The listing builds one solid part. Answer for the finished solid, in the listing's coordinates (mm). A direction names the side the tool comes from. Give positions to 0.01 mm unless a question says otherwise; leave off trailing zeros. Order: outer loops, then holes, each group sorted by start corner. A loop starts at its lowest first (then second) coordinate and runs counter-clockwise, first axis right, second up. Notation, with made-up numbers: (70, 58.5) - (92, 58.5) arc R20 ccw to (92, 96.5) - close; hole circle Ø6 at (-19, 32). An arc over 180 degrees is marked (long way). Answer as a JSON object with one key per item and string values. Group by question number.
Q1. A cutting plane is placed at A-A, the plane z = -4. Give the vertices of the cut face in (x, y).
Q2. A cutting plane is placed at D-D, the plane y = 63.5. Give the vertices of the cut face in (x, z) (3 decimals).
Q3. Consider line 1 (Z direction, x = 0, y = -69); line 2 (Y direction, x = 4.5, z = -7); line 3 (Y direction, x = 3, z = 4). Determine where each line is inside the solid, lowest interval first.
Q4. For faces 1 (the face through (5.21, -69.94, 1.64)), 2 (the face through (3, -76.2, 5)), determine the directions among +Z, -Z, +X, -X, +Y, -Y from which every point of the face is accessible in a straight line to the end or side of a thin tool.
Q5. Given pin 1 (2 mm diameter, centred on x = 1.5, y = -13.5, fed in from +Z); pin 2 (5 mm diameter, centred on y = -56, z = 7, fed in from +X); pin 3 (3.5 mm diameter, centred on x = -2, z = 2, fed in from -Y), each flat-ended and moving along its own axis, determine where each tip first touches the part or whether it passes through.
Q6. The mould has two halves that part along Z. Classify faces 3 (the face through (8.98, 46.96, 2.76)), 4 (the face through (1.9, 0, -6.3)), 5 (the face through (0, -63.5, 0)): released by +Z, released by -Z, zero draft, split by the parting line, or undercut.
Q7. A cutting plane is placed at B-B, the plane x = 4. Give the vertices of the cut face in (y, z).
Q8. A cutting plane is placed at C-C, the plane y = -58. Give the vertices of the cut face in (x, z).
from build123d import *

# Parameters (mm, degrees)
F0_R     = 9.525
F1_DEPTH = 95.25
F2_R     = 6.35
F3_DEPTH = 76.2
F4_R     = 5.461
F5_DEPTH = 12.7


with BuildPart() as f1:
    # F0 (on Front) → F1 (new body)
    with BuildSketch(Plane.XZ):
        with Locations((-0.102708, -0.103876)):
            Circle(F0_R)
    extrude(amount=-F1_DEPTH)

    # F2 (on face) → F3 (join)
    with BuildSketch(Plane.XZ):
        Circle(F2_R)
    extrude(amount=F3_DEPTH)

    # F4 (on face) → F5 (cut)
    with BuildSketch(Plane.XZ.offset(76.2)):
        Circle(F4_R)
    extrude(amount=-F5_DEPTH, mode=Mode.SUBTRACT)


solid = f1.part
Reply:
{
 "1": {"outline": "(-8.79, 0) - (-4.93, 0) - (-4.93, -76.2) - (-3.72, -76.2) - (-3.72, -63.5) - (3.72, -63.5) - (3.72, -76.2) - (4.93, -76.2) - (4.93, 0) - (8.59, 0) - (8.59, 95.25) - (-8.79, 95.25) - close"},
 "2": {"outline": "circle Ø19.05 at (-0.103, -0.104)"},
 "3": {"line 1": "z = -6.35 to -5.46, 5.46 to 6.35", "line 2": "y = 0 to 95.25", "line 3": "y = -63.5 to 95.25"},
 "4": {"face 1": "-Y", "face 2": "+Z, -Z, +X, -X, -Y"},
 "5": {"pin 1": "stops at z = 6.33", "pin 2": "stops at x = 4.48", "pin 3": "stops at y = -63.5"},
 "6": {"face 3": "split by the parting line", "face 4": "zero draft", "face 5": "undercut"},
 "7": {"outline": "(-76.2, -4.93) - (0, -4.93) - (0, -8.7) - (95.25, -8.7) - (95.25, 8.49) - (0, 8.49) - (0, 4.93) - (-76.2, 4.93) - (-76.2, 3.72) - (-63.5, 3.72) - (-63.5, -3.72) - (-76.2, -3.72) - close"},
 "8": {"outline": "circle Ø12.7 at (0, 0)"}
}
